Check sheet for the modelled part. Datum: model origin and axes. Units: mm. A direction names the side the tool comes from. Give positions to 0.01 mm unless a question says otherwise; leave off trailing zeros. Write each loop counter-clockwise with the first axis right and the second up, starting at its lowest first coordinate (ties: lowest second). Pieces come first, ordered by that corner, then holes. Notation, with made-up numbers: M -11.5,10.5 L -1.5,10.5 A21 ccw -1.5,32.5 Z; hole C -14,77.5 d5. An arc over 180 degrees is marked long. Use CSV: the item, a comma, the result in double quotes. Start each with the question number.
1. Scan lines: line 1 (Y direction, x = -4.5, z = -5) (3 decimals); line 2 (Y direction, x = -3, z = 0.5); line 3 (X direction, y = -1.5, z = 13.5). Record each from-to range of solid material in increasing order.
2. Depth check by flat-ended pin: P1, Ø2.5, axis at x = -1, z = 6.5, coming from the +Y side; P2, Ø3, axis at y = 11.875, z = -5, coming from the +X side; P3, Ø2.5, axis at x = -2, y = 16.5, coming from the -Z side; P4, Ø1, axis at x = -1, z = 15, coming from the -Y side. Enter the tip coordinate at first touch or a pass-through.
3. Cross-section at B-B, the plane y = 5. Enter the section's corners in (x, z), and give its area (3 significant figures).
4. Cross-section at D-D, the plane x = -2.75. Enter the section's corners in (y, z).
5. Mould release check, pull along Y, two halves, no side actions. Record for faces 5 (the face through (-5.02, 11.96, -6.9)), 6 (the face through (-8, 0, 12)), 7 (the face through (-3.35, 12, -1)): +Y half, -Y half, draft (parallel to the pull), parting line (faces both ways), or undercut.
6. Access from +Z, -Z, +X, -X, +Y, -Y to the whole of each face (thin tool, end or side, straight path). Record for faces 1 (the face through (-2, 12, 0)), 2 (the face through (-8, 12, 0)), 3 (the face through (-2, 23.75, 12)), 4 (the face through (-8, 23.75, 12)).
7. Cross-section at C-C, the plane z = 16.5. Enter the section's corners in (x, y), and give its area (3 significant figures).
8. Cross-section at A-A, the plane z = -5. Enter the section's corners in (x, y) (3 decimals).
from build123d import *

# Parameters (mm, degrees)
SKETCH1_W           = 23.75
SKETCH1_H           = 24
BOSS_EXTRUDE1_DEPTH = 10
SKETCH2_W           = 3.3
SKETCH2_H           = 9.8
BOSS_EXTRUDE2_DEPTH = 23.75
SKETCH3_W           = 3.3
SKETCH3_H           = 33.8
BOSS_EXTRUDE3_DEPTH = 4.9
CUT_EXTRUDE1_REACH  = 36.413
SKETCH4_R           = 1.9


with BuildPart() as part:
    # Sketch1 → Boss-Extrude1 (new body)
    with BuildSketch(Plane.YZ):
        with Locations((11.875, 12)):
            Rectangle(SKETCH1_W, SKETCH1_H)
    extrude(amount=-BOSS_EXTRUDE1_DEPTH)

    # Sketch2 → Boss-Extrude2 (add, through all)
    with BuildSketch(Plane.XZ):
        with Locations((-5, -4.9)):
            Rectangle(SKETCH2_W, SKETCH2_H)
    extrude(amount=-BOSS_EXTRUDE2_DEPTH)

    # Sketch3 → Boss-Extrude3 (add)
    with BuildSketch(Plane.XZ):
        with Locations((-5, 7.1)):
            Rectangle(SKETCH3_W, SKETCH3_H)
    boss_extrude3 = extrude(amount=BOSS_EXTRUDE3_DEPTH)

    # Sketch4 → Cut-Extrude1 (cut, up to next)
    with BuildSketch(Plane(origin=(-6.65, 0, 0), x_dir=(0, -1, 0), z_dir=(-1, 0, 0)), mode=Mode.PRIVATE) as cut_extrude1_sk1:
        with Locations(Location((-11.875, -5, 0), (0, 0, 90))):
            Circle(SKETCH4_R)
    cut_extrude1_tool1 = extrude(cut_extrude1_sk1.sketch, amount=-CUT_EXTRUDE1_REACH, mode=Mode.PRIVATE) & part.part
    add(cut_extrude1_tool1.solids().sort_by_distance((-6.65, 11.875, -5))[0], mode=Mode.SUBTRACT)

    # Mirror1: Boss-Extrude3 across plane
    add(boss_extrude3.mirror(Plane(origin=(0, 11.875, 0), x_dir=(0, 0, 1), z_dir=(0, -1, 0))))


solid = part.part
Worked answers:
1,line 1,"y = -4.9 to 9.975, 13.775 to 28.65"
1,line 2,"y = 0 to 23.75"
1,line 3,"x = -6.65 to -3.35"
2,P1,"stops at y = 23.75"
2,P2,"passes through"
2,P3,"stops at z = 0"
2,P4,"stops at y = 0"
3,outline,"M -10,0 L -6.65,0 L -6.65,-9.8 L -3.35,-9.8 L -3.35,0 L 0,0 L 0,24 L -10,24 Z"
3,area,"272 mm^2"
4,outline,"M 0,0 L 23.75,0 L 23.75,24 L 0,24 Z"
5,face 5,"undercut"
5,face 6,"-Y half"
5,face 7,"draft"
6,face 1,"-Z, +X, +Y, -Y"
6,face 2,"-Z, -X, +Y, -Y"
6,face 3,"+Z, -Z, +X, +Y"
6,face 4,"+Z, -Z, -X, +Y"
7,outline,"M -10,0 L -6.65,0 L -6.65,-4.9 L -3.35,-4.9 L -3.35,0 L 0,0 L 0,23.75 L -3.35,23.75 L -3.35,28.65 L -6.65,28.65 L -6.65,23.75 L -10,23.75 Z"
7,area,"270 mm^2"
8,outline,"M -6.65,-4.9 L -3.35,-4.9 L -3.35,9.975 L -6.65,9.975 Z; M -6.65,13.775 L -3.35,13.775 L -3.35,28.65 L -6.65,28.65 Z"
